The model under review builds one solid part; all positions refer to its coordinate system, in mm. A direction names the side the tool comes from. Round coordinates to 2 decimals unless told otherwise and drop trailing zeros. Loops run counter-clockwise (first coordinate to the right, second up) from the corner with the lowest first, then second, coordinate; pieces in that order, holes last. Notation, with made-up numbers: M 39,-13.75 L 64,-13.75 A17 ccw 64,1.25 Z; hole C -39,45 d2. An arc over 180 degrees is marked long. Return JSON: item names as keys, results as strings. Group by question number.
Q1. Consider section A-A (z = 7). State the section outline as (x, y) points, and give its area (3 significant figures).
Q2. Consider section C-C (y = -16). State the section outline as (x, z) points.
Q3. To check wall thickness, follow line 1 along Y through (x, z) = (28, 2.25); line 2 along Y through (x, z) = (-27.5, 7); line 3 along Z through (x, y) = (13.5, -2). State the ranges of each line that lie inside material, in increasing order.
Q4. For faces 1 (the face through (-17, 3.775, 1)), 2 (the face through (0, 19, 1)), 3 (the face through (-5.5, 0, 13)), list the 3-axis set-ups (+Z, -Z, +X, -X, +Y, -Y) from which the entire face can be reached by the end or side of a thin tool; tool diameter is ignored.
Q5. Consider section B-B (z = 1.5). State the section outline as (x, y) points, and give its area (3 significant figures).
Q6. Draft analysis for pull direction Y (two halves, no side actions). For faces 4 (the face through (28.5, 0, 1)), 5 (the face through (-28.5, 3, 12)), 6 (the face through (23.077, -6.674, 3.783)), 7 (the face through (23, 3.775, 1)), state which applies: pulls with the +Y half, pulls with the -Y half, needs draft (parallel to the pull), parting line crosses it, or undercut.
Q7. Clearance check with flat-ended pins moving along their axes: pin 1 Ø1.5 at (y, z) = (14, 5.5) entering from +X; pin 2 Ø5.5 at (y, z) = (3.5, 8.5) entering from -X; pin 3 Ø2 at (x, y) = (25.5, -4) entering from +Z; pin 4 Ø1.5 at (x, y) = (21, 0.5) entering from -Z. State where each tip first meets the part, or that it passes through.
Q8. Consider section D-D (x = -26). State the section outline as (y, z) points, and give its area (3 significant figures).
from build123d import *

# Parameters (mm, degrees)
SKETCH1_W           = 71
SKETCH1_H           = 38
SKETCH1_R           = 3.7499999999999996
SKETCH1_R_2         = 3.750000000000006
BOSS_EXTRUDE1_DEPTH = 3
SKETCH3_R           = 6.500000000000002
SKETCH3_R_2         = 5.5
BOSS_EXTRUDE2_DEPTH = 18
BOSS_EXTRUDE3_START = -30
SKETCH4_R           = 6.500000000000001
SKETCH4_R_2         = 5.499999999999999
BOSS_EXTRUDE3_DEPTH = 30
SKETCH5_W           = 11
SKETCH5_H           = 7.54983443527075
CUT_EXTRUDE2_DEPTH  = 30
CUT_EXTRUDE3_START  = -7
CUT_EXTRUDE3_DEPTH  = 7
CUT_EXTRUDE4_DEPTH  = 7
FILLET2_R           = 2
FILLET3_R           = 2


with BuildPart() as part:
    # Sketch1 → Boss-Extrude1 (new body)
    with BuildSketch(Plane.XY):
        Rectangle(SKETCH1_W, SKETCH1_H)
        with Locations((-27.999999999999996, 13.000000000000004)):
            Circle(SKETCH1_R, mode=Mode.SUBTRACT)
        with Locations((27.999999999999996, 13)):
            Circle(SKETCH1_R, mode=Mode.SUBTRACT)
        with Locations((-27.999999999999996, -12.999999999999996)):
            Circle(SKETCH1_R, mode=Mode.SUBTRACT)
        with Locations((27.999999999999996, -12.999999999999996)):
            Circle(SKETCH1_R_2, mode=Mode.SUBTRACT)
    extrude(amount=BOSS_EXTRUDE1_DEPTH)

    # Sketch3 → Boss-Extrude2 (add)
    with BuildSketch(Plane(origin=(35.5, 0, 0), x_dir=(0, 0, -1), z_dir=(1, 0, 0))):
        with Locations((-7, 3.47e-15)):
            Circle(SKETCH3_R)
        with Locations((-7, 3.47e-15)):
            Circle(SKETCH3_R_2, mode=Mode.SUBTRACT)
    extrude(amount=-BOSS_EXTRUDE2_DEPTH)

    # Sketch4 → Boss-Extrude3 (add)
    with BuildSketch(Plane.ZY.offset(35.5).offset(BOSS_EXTRUDE3_START)):
        with Locations((7, 3.47e-15)):
            Circle(SKETCH4_R)
        with Locations((7, 3.47e-15)):
            Circle(SKETCH4_R_2, mode=Mode.SUBTRACT)
    extrude(amount=BOSS_EXTRUDE3_DEPTH)

    # Sketch5 → Cut-Extrude2 (cut)
    with BuildSketch(Plane.XY.offset(3)):
        Polygon((-5.499999999999998, 3.7749172176353767), (-28.499999999999996, 3.7749172176353745), (-28.499999999999996, -3.77491721763537), (-5.499999999999998, -3.77491721763537), align=None)
        with Locations((22.999999999999996, 3.33e-15)):
            Rectangle(SKETCH5_W, SKETCH5_H)
    extrude(amount=-CUT_EXTRUDE2_DEPTH, mode=Mode.SUBTRACT)

    # Sketch6 → Cut-Extrude3 (cut)
    with BuildSketch(Plane.ZY.offset(35.5).offset(CUT_EXTRUDE3_START)):
        with BuildLine():
            Line((3, 3.7749172176353767), (3, 5.123475382979803))
            ThreePointArc((3, 5.123475382979803), (13.5, 6.36e-15), (3, -5.123475382979797))
            Line((3, -5.123475382979797), (3, -3.77491721763537))
            ThreePointArc((3, -3.77491721763537), (12.5, 3.47e-15), (3, 3.7749172176353767))
        make_face()
    extrude(amount=CUT_EXTRUDE3_DEPTH, mode=Mode.SUBTRACT)

    # Sketch7 → Cut-Extrude4 (cut)
    with BuildSketch(Plane(origin=(35.5, 0, 0), x_dir=(0, 0, -1), z_dir=(1, 0, 0))):
        with BuildLine():
            Line((-3, 5.123475382979803), (-3, 3.774917217635378))
            ThreePointArc((-3, 3.774917217635378), (-12.5, 4.14e-15), (-3, -3.774917217635371))
            Line((-3, -3.774917217635371), (-3, -5.123475382979797))
            ThreePointArc((-3, -5.123475382979797), (-13.5, 4.27e-15), (-3, 5.123475382979803))
        make_face()
    extrude(amount=-CUT_EXTRUDE4_DEPTH, mode=Mode.SUBTRACT)

    # Fillet2
    fillet2_edges = [part.edges().sort_by_distance(p)[0] for p in [
        (-17, 5.123475382979804, 3),
        (23, -5.123475382979798, 3),
        (23, 5.123475382979805, 3),
        (-17, -5.123475382979797, 3),
    ]]
    fillet(fillet2_edges, radius=FILLET2_R)

    # Fillet3
    # the kernel refuses this fillet: 2 mm, written as the material it takes off along each edge
    with BuildSketch(Plane(origin=(17.5, 3.7749172176353785, 3), x_dir=(0, 0, -1), z_dir=(1, 0, 0))) as fillet3_piece_1:
        with BuildLine():
            CenterArc((0.7854290434049434, 2), FILLET3_R, 230.35289769223547, 39.6471023077645)
            ThreePointArc((-0.49068536816965125, 0.460022075297303), (-0.2383040211369254, 0.23751887065380473), (0, 0))
            Line((0, 0), (0.7854290434049434, 0))
        make_face()
    extrude(amount=10.999999999999996, mode=Mode.SUBTRACT)
    with BuildSketch(Plane(origin=(-28.499999999999996, -3.77491721763537, 3), x_dir=(0, 5.7e-16, -1), z_dir=(1, 0, 0))) as fillet3_piece_2:
        with BuildLine():
            CenterArc((0.7854290434049418, -2), FILLET3_R, 89.99999999999997, 39.64710230776453)
            ThreePointArc((-0.49068536816965286, -0.46002207529730227), (-0.23830402113692464, -0.23751887065380414), (0, 0))
            Line((0, 0), (0.7854290434049429, 0))
        make_face()
    extrude(amount=22.999999999999996, mode=Mode.SUBTRACT)
    with BuildSketch(Plane(origin=(17.5, -3.7749172176353714, 3), x_dir=(0, -0.6839447234296507, 0.7295338342343956), z_dir=(1, 0, 0))) as fillet3_piece_3:
        with BuildLine():
            CenterArc((0.7948923853050224, 1.9962577183336636), FILLET3_R, 226.84732795972278, 39.647102307770695)
            Line((-0.572997061554437, 0.5371900498650203), (0, 0))
            ThreePointArc((0, 0), (0.33630062455212534, 0.01029127458242615), (0.6726012491042509, 1e-17))
        make_face()
    extrude(amount=10.999999999999996, mode=Mode.SUBTRACT)
    with BuildSketch(Plane(origin=(-28.499999999999996, 3.774917217635377, 3), x_dir=(0, 0.6839447234296516, 0.7295338342343948), z_dir=(1, 0, 0))) as fillet3_piece_4:
        with BuildLine():
            CenterArc((0.7948923853050189, -1.9962577183336638), FILLET3_R, 93.50556973250654, 39.647102307770794)
            Line((-0.5729970615544441, -0.5371900498650239), (0, 0))
            ThreePointArc((0, 0), (0.3363006245521229, -0.01029127458242505), (0.6726012491042468, -6e-17))
        make_face()
    extrude(amount=22.999999999999996, mode=Mode.SUBTRACT)


solid = part.part
Values:
{
 "1": {"outline": "M -28.5,-6.5 L -5.5,-6.5 L -5.5,-5.5 L -28.5,-5.5 Z; M -28.5,5.5 L -5.5,5.5 L -5.5,6.5 L -28.5,6.5 Z; M 17.5,-6.5 L 28.5,-6.5 L 28.5,-5.5 L 17.5,-5.5 Z; M 17.5,5.5 L 28.5,5.5 L 28.5,6.5 L 17.5,6.5 Z", "area": "68.0 mm2"},
 "2": {"outline": "M -35.5,0 L -30.25,0 L -30.25,3 L -35.5,3 Z; M -25.75,0 L 25.75,0 L 25.75,3 L -25.75,3 Z; M 30.25,0 L 35.5,0 L 35.5,3 L 30.25,3 Z"},
 "3": {"line 1": "y = -19 to -16.75, -9.25 to -3.78, 3.78 to 9.25, 16.75 to 19", "line 2": "y = -6.5 to -5.5, 5.5 to 6.5", "line 3": "z = 0 to 3"},
 "4": {"face 1": "-Z", "face 2": "+Z, -Z, +X, -X, +Y", "face 3": "+Z, +Y, -Y"},
 "5": {"outline": "M -35.5,-19 L 35.5,-19 L 35.5,19 L -35.5,19 Z; hole C -28,-13 d7.5; hole C -28,13 d7.5; hole M -28.5,-3.77 L -5.5,-3.77 L -5.5,3.77 L -28.5,3.77 Z; hole M 17.5,-3.77 L 28.5,-3.77 L 28.5,3.77 L 17.5,3.77 Z; hole C 28,-13 d7.5; hole C 28,13 d7.5", "area": "2,260 mm2"},
 "6": {"face 4": "undercut", "face 5": "needs draft", "face 6": "pulls with the -Y half", "face 7": "undercut"},
 "7": {"pin 1": "passes through", "pin 2": "stops at x = -28.5", "pin 3": "stops at z = 12.77", "pin 4": "stops at z = 12.36"},
 "8": {"outline": "M -19,0 L -16.17,0 L -16.17,3 L -19,3 Z; M -9.83,0 L -3.77,0 L -3.77,2.21 A2 ccw -4.23,3.49 A5.5 cw long 4.23,3.49 A2 ccw 3.77,2.21 L 3.77,0 L 9.83,0 L 9.83,3 L 8.26,3 A2 cw 6.32,5.47 A6.5 ccw long -6.32,5.47 A2 cw -8.26,3 L -9.83,3 Z; M 16.17,0 L 19,0 L 19,3 L 16.17,3 Z", "area": "84.6 mm2"}
}
